```python
from build123d import *

# Parameters (mm, degrees)
SKETCH1_W                = 42
SKETCH1_H                = 14
BOSS_EXTRUDE1_DEPTH      = 20
SKETCH2_W                = 11
SKETCH2_H                = 10
CUT_EXTRUDE1_DEPTH       = 33.202484376
SKETCH3_W                = 11
SKETCH3_H                = 10
CUT_EXTRUDE2_DEPTH       = 33.202484376
SKETCH4_W                = 12
SKETCH4_H                = 10
CUT_EXTRUDE3_DEPTH       = 33.202484376
F_4_0_4_DIAMETER_HOLE1_D = 4
FILLET1_R                = 1
SKETCH7_W                = 53.135320533
SKETCH7_H                = 18.013507302
CUT_EXTRUDE4_DEPTH       = 1.5
SKETCH8_W                = 12
SKETCH8_H                = 12.5
CUT_EXTRUDE5_DEPTH       = 1.5
SKETCH9_W                = 20
SKETCH9_H                = 20
BOSS_EXTRUDE2_DEPTH      = 1
SKETCH10_W               = 3.48641985
SKETCH10_H               = 13.666765812
CUT_EXTRUDE6_DEPTH       = 3
SKETCH11_W               = 4.358024812
SKETCH11_H               = 13.509876918
CUT_EXTRUDE7_DEPTH       = 3
BOSS_EXTRUDE3_START      = 0.5
SKETCH14_W               = 12
SKETCH14_H               = 12.5
SKETCH14_R               = 2
BOSS_EXTRUDE3_DEPTH      = 0.5
FILLET7_R                = 3
BOSS_EXTRUDE4_START      = -14
SKETCH15_W               = 4
SKETCH15_H               = 20
BOSS_EXTRUDE4_DEPTH      = 14
SKETCH16_W               = 13.925462325
SKETCH16_H               = 21.292387115
SKETCH16_W_2             = 9.897316219
SKETCH16_H_2             = 21.744987801
CUT_EXTRUDE8_DEPTH       = 30.241451742
SKETCH17_W               = 12
SKETCH17_H               = 7.5
CUT_EXTRUDE9_DEPTH       = 1.5
SKETCH18_W               = 29.147036291
SKETCH18_H               = 2.174846481
CUT_EXTRUDE10_DEPTH      = 5.897378098
SKETCH19_W               = 12
SKETCH19_H               = 20
BOSS_EXTRUDE5_DEPTH      = 1.5
SKETCH20_W               = 4
SKETCH20_H               = 1.602621902
BOSS_EXTRUDE6_DEPTH      = 1.5
SKETCH24_R               = 1.75
CUT_EXTRUDE11_DEPTH      = 14
SKETCH25_R               = 3.5
CUT_EXTRUDE12_DEPTH      = 1
FILLET8_R                = 2


with BuildPart() as part:
    # Sketch1 → Boss-Extrude1 (new body)
    with BuildSketch(Plane.XZ.offset(6.25)):
        with Locations((0, 7)):
            Rectangle(SKETCH1_W, SKETCH1_H)
    extrude(amount=-BOSS_EXTRUDE1_DEPTH)

    # Sketch2 → Cut-Extrude1 (cut, through all)
    with BuildSketch(Plane(origin=(0, 13.75, 0), x_dir=(-1, 0, 0), z_dir=(0, 1, 0))):
        with Locations((-15.5, 9)):
            Rectangle(SKETCH2_W, SKETCH2_H)
    extrude(amount=-CUT_EXTRUDE1_DEPTH, mode=Mode.SUBTRACT)

    # Sketch3 → Cut-Extrude2 (cut, through all)
    with BuildSketch(Plane(origin=(0, 13.75, 0), x_dir=(-1, 0, 0), z_dir=(0, 1, 0))):
        with Locations((15.5, 9)):
            Rectangle(SKETCH3_W, SKETCH3_H)
    extrude(amount=-CUT_EXTRUDE2_DEPTH, mode=Mode.SUBTRACT)

    # Sketch4 → Cut-Extrude3 (cut, through all)
    with BuildSketch(Plane(origin=(0, 13.75, 0), x_dir=(-1, 0, 0), z_dir=(0, 1, 0))):
        with Locations((0, 5)):
            Rectangle(SKETCH4_W, SKETCH4_H)
    extrude(amount=-CUT_EXTRUDE3_DEPTH, mode=Mode.SUBTRACT)

    # Ø4.0 (4) Diameter Hole1 (through all)
    with Locations(Plane.XY.offset(4)):
        with Locations((15, 0), (-15, 0)):
            Hole(F_4_0_4_DIAMETER_HOLE1_D / 2)

    # Fillet1
    fillet1_edges = [part.edges().sort_by_distance(p)[0] for p in [
        (-21, -6.25, 2),
        (-21, 13.75, 2),
        (21, -6.25, 2),
        (21, 13.75, 2),
    ]]
    fillet(fillet1_edges, radius=FILLET1_R)

    # Sketch7 → Cut-Extrude4 (cut)
    with BuildSketch(Plane(origin=(0, 0, 0), x_dir=(-1, 0, 0), z_dir=(0, 0, -1))):
        with Locations((2.896644391, -1.154131749)):
            Rectangle(SKETCH7_W, SKETCH7_H)
    extrude(amount=-CUT_EXTRUDE4_DEPTH, mode=Mode.SUBTRACT)

    # Sketch8 → Cut-Extrude5 (cut)
    with BuildSketch(Plane(origin=(0, 0, 10), x_dir=(-1, 0, 0), z_dir=(0, 0, -1))):
        Rectangle(SKETCH8_W, SKETCH8_H)
    extrude(amount=-CUT_EXTRUDE5_DEPTH, mode=Mode.SUBTRACT)

    # Sketch9 → Boss-Extrude2 (add)
    with BuildSketch(Plane.XY.offset(14)):
        with Locations((0, 3.75)):
            Rectangle(SKETCH9_W, SKETCH9_H)
    extrude(amount=BOSS_EXTRUDE2_DEPTH)

    # Sketch10 → Cut-Extrude6 (cut)
    with BuildSketch(Plane.ZY.offset(21)):
        with Locations((2.776320836, -0.252765439)):
            Rectangle(SKETCH10_W, SKETCH10_H)
    extrude(amount=-CUT_EXTRUDE6_DEPTH, mode=Mode.SUBTRACT)

    # Sketch11 → Cut-Extrude7 (cut)
    with BuildSketch(Plane(origin=(21, 0, 0), x_dir=(0, 0, -1), z_dir=(1, 0, 0))):
        with Locations((-2.462543049, -0.261481489)):
            Rectangle(SKETCH11_W, SKETCH11_H)
    extrude(amount=-CUT_EXTRUDE7_DEPTH, mode=Mode.SUBTRACT)

    # Sketch14 → Boss-Extrude3 (add)
    # profile 1 of 2: a face of its own
    with BuildSketch(Plane(origin=(0, 0, 1.5), x_dir=(-1, 0, 0), z_dir=(0, 0, -1)).offset(BOSS_EXTRUDE3_START)):
        with Locations((12, 0)):
            Rectangle(SKETCH14_W, SKETCH14_H)
        with Locations(Location((15, 0, 0), (0, 0, 180))):
            Circle(SKETCH14_R, mode=Mode.SUBTRACT)
    # profile 2 of 2: a face of its own
    with BuildSketch(Plane(origin=(0, 0, 1.5), x_dir=(-1, 0, 0), z_dir=(0, 0, -1)).offset(BOSS_EXTRUDE3_START)):
        with Locations((-12, 0)):
            Rectangle(SKETCH14_W, SKETCH14_H)
        with Locations(Location((-15, 0, 0), (0, 0, 180))):
            Circle(SKETCH14_R, mode=Mode.SUBTRACT)
    extrude(amount=-BOSS_EXTRUDE3_DEPTH)

    # Fillet7
    # the kernel refuses this fillet: 3 mm, written as the material it takes off along each edge
    with BuildSketch(Plane(origin=(-18, -6.25, 1.5), x_dir=(1, 0, 0), z_dir=(0, 0, 1))) as fillet7_piece_1:
        with BuildLine():
            CenterArc((FILLET7_R, FILLET7_R), FILLET7_R, 180, 90)
            Line((0, FILLET7_R), (0, 0))
            Line((0, 0), (FILLET7_R, 0))
        make_face()
    extrude(amount=10, mode=Mode.SUBTRACT)
    with BuildSketch(Plane(origin=(18, -6.25, 11.5), x_dir=(-1, 0, 0), z_dir=(0, 0, -1))) as fillet7_piece_2:
        with BuildLine():
            CenterArc((FILLET7_R, FILLET7_R), FILLET7_R, 180, 90)
            Line((0, FILLET7_R), (0, 0))
            Line((0, 0), (FILLET7_R, 0))
        make_face()
    extrude(amount=18, mode=Mode.SUBTRACT)
    with BuildSketch(Plane(origin=(-18, 6.25, -6.5), x_dir=(1, 0, 0), z_dir=(0, 0, 1))) as fillet7_piece_3:
        with BuildLine():
            CenterArc((FILLET7_R, -FILLET7_R), FILLET7_R, 90, 90)
            Line((0, -FILLET7_R), (0, 0))
            Line((0, 0), (FILLET7_R, 0))
        make_face()
    extrude(amount=8, mode=Mode.SUBTRACT)
    with BuildSketch(Plane(origin=(-18, -6.25, -6.5), x_dir=(1, 0, 0), z_dir=(0, 0, 1))) as fillet7_piece_4:
        with BuildLine():
            CenterArc((FILLET7_R, FILLET7_R), FILLET7_R, 180, 90)
            Line((0, FILLET7_R), (0, 0))
            Line((0, 0), (FILLET7_R, 0))
        make_face()
    extrude(amount=8, mode=Mode.SUBTRACT)

    # Sketch15 → Boss-Extrude4 (add)
    with BuildSketch(Plane.XY.offset(15).offset(BOSS_EXTRUDE4_START)):
        with Locations((-12, 3.75)):
            Rectangle(SKETCH15_W, SKETCH15_H)
        with Locations((12, 3.75)):
            Rectangle(SKETCH15_W, SKETCH15_H)
    extrude(amount=BOSS_EXTRUDE4_DEPTH)

    # Sketch16 → Cut-Extrude8 (cut, through all)
    with BuildSketch(Plane.XY.offset(15)):
        with Locations((20.962731162, 3.103806442)):
            Rectangle(SKETCH16_W, SKETCH16_H)
        with Locations((-18.94865811, 2.877506099)):
            Rectangle(SKETCH16_W_2, SKETCH16_H_2)
    extrude(amount=-CUT_EXTRUDE8_DEPTH, mode=Mode.SUBTRACT)

    # Sketch17 → Cut-Extrude9 (cut)
    with BuildSketch(Plane(origin=(0, 0, 10), x_dir=(-1, 0, 0), z_dir=(0, 0, -1))):
        with Locations((0, 10)):
            Rectangle(SKETCH17_W, SKETCH17_H)
    extrude(amount=-CUT_EXTRUDE9_DEPTH, mode=Mode.SUBTRACT)

    # Sketch18 → Cut-Extrude10 (cut)
    with BuildSketch(Plane(origin=(0, 7.852621902, 0), x_dir=(-1, 0, 0), z_dir=(0, -1, 0))):
        with Locations((-0.573518146, 0.087423241)):
            Rectangle(SKETCH18_W, SKETCH18_H)
    extrude(amount=-CUT_EXTRUDE10_DEPTH, mode=Mode.SUBTRACT)

    # Sketch19 → Boss-Extrude5 (add)
    with BuildSketch(Plane(origin=(0, 0, 11.5), x_dir=(-1, 0, 0), z_dir=(0, 0, -1))):
        with Locations((0, 3.75)):
            Rectangle(SKETCH19_W, SKETCH19_H)
    extrude(amount=BOSS_EXTRUDE5_DEPTH)

    # Sketch20 → Boss-Extrude6 (add)
    with BuildSketch(Plane(origin=(0, 0, 1), x_dir=(-1, 0, 0), z_dir=(0, 0, -1))):
        with Locations((-8, 7.051310951)):
            Rectangle(SKETCH20_W, SKETCH20_H)
        with Locations((8, 7.051310951)):
            Rectangle(SKETCH20_W, SKETCH20_H)
    extrude(amount=-BOSS_EXTRUDE6_DEPTH)

    # Sketch24 → Cut-Extrude11 (cut)
    with BuildSketch(Plane(origin=(0, 0, 1), x_dir=(-1, 0, 0), z_dir=(0, 0, -1))):
        with Locations((-10, 5.75)):
            Circle(SKETCH24_R)
        with Locations((10, 5.75)):
            Circle(SKETCH24_R)
    extrude(amount=-CUT_EXTRUDE11_DEPTH, mode=Mode.SUBTRACT)

    # Sketch25 → Cut-Extrude12 (cut)
    with BuildSketch(Plane.XY.offset(15)):
        with Locations((10, 5.75)):
            Circle(SKETCH25_R)
        with Locations((-10, 5.75)):
            Circle(SKETCH25_R)
    extrude(amount=-CUT_EXTRUDE12_DEPTH, mode=Mode.SUBTRACT)

    # Fillet8
    # the kernel refuses this fillet: 2 mm, written as the material it takes off along each edge
    with BuildSketch(Plane(origin=(12, -4.25, 13), x_dir=(0, 0, 1), z_dir=(1, 0, 0))) as fillet8_piece_1_section:
        Polygon((0, 0), (FILLET8_R, 0), (FILLET8_R, FILLET8_R), (0, FILLET8_R), align=None)
    fillet8_piece_1 = extrude(amount=FILLET8_R, mode=Mode.PRIVATE)
    fillet8_piece_1 = fillet8_piece_1 - Plane(origin=(12, -4.25, 13), x_dir=(0, 0.7071067811865475, -0.7071067811865475), z_dir=(1, 0, 0)) * Sphere(FILLET8_R, mode=Mode.PRIVATE)
    add(fillet8_piece_1, mode=Mode.SUBTRACT)
    with BuildSketch(Plane(origin=(-12, -4.25, 13), x_dir=(0, -1, 0), z_dir=(0, 0, 1))) as fillet8_piece_2_section:
        Polygon((0, 0), (FILLET8_R, 0), (FILLET8_R, -FILLET8_R), (0, -FILLET8_R), align=None)
    fillet8_piece_2 = extrude(amount=FILLET8_R, mode=Mode.PRIVATE)
    fillet8_piece_2 = fillet8_piece_2 - Plane(origin=(-12, -4.25, 13), x_dir=(0.7071067811865475, 0.7071067811865475, 0), z_dir=(0, 0, 1)) * Sphere(FILLET8_R, mode=Mode.PRIVATE)
    add(fillet8_piece_2, mode=Mode.SUBTRACT)
    with BuildSketch(Plane(origin=(-12, 11.75, 13), x_dir=(0, 0, 1), z_dir=(0, 1, 0))) as fillet8_piece_3_section:
        Polygon((0, 0), (FILLET8_R, 0), (FILLET8_R, -FILLET8_R), (0, -FILLET8_R), align=None)
    fillet8_piece_3 = extrude(amount=FILLET8_R, mode=Mode.PRIVATE)
    fillet8_piece_3 = fillet8_piece_3 - Plane(origin=(-12, 11.75, 13), x_dir=(0.7071067811865475, 0, -0.7071067811865475), z_dir=(0, 1, 0)) * Sphere(FILLET8_R, mode=Mode.PRIVATE)
    add(fillet8_piece_3, mode=Mode.SUBTRACT)
    with BuildSketch(Plane(origin=(12, 11.75, 13), x_dir=(0, 1, 0), z_dir=(1, 0, 0))) as fillet8_piece_4_section:
        Polygon((0, 0), (FILLET8_R, 0), (FILLET8_R, FILLET8_R), (0, FILLET8_R), align=None)
    fillet8_piece_4 = extrude(amount=FILLET8_R, mode=Mode.PRIVATE)
    fillet8_piece_4 = fillet8_piece_4 - Plane(origin=(12, 11.75, 13), x_dir=(0, -0.7071067811865475, -0.7071067811865475), z_dir=(1, 0, 0)) * Sphere(FILLET8_R, mode=Mode.PRIVATE)
    add(fillet8_piece_4, mode=Mode.SUBTRACT)
    with BuildSketch(Plane(origin=(12, -6.25, 15), x_dir=(0, 1, 0), z_dir=(-1, 0, 0))) as fillet8_piece_5:
        with BuildLine():
            CenterArc((FILLET8_R, FILLET8_R), FILLET8_R, 180, 90)
            Line((0, FILLET8_R), (0, 0))
            Line((0, 0), (FILLET8_R, 0))
        make_face()
    extrude(amount=24, mode=Mode.SUBTRACT)
    with BuildSketch(Plane(origin=(-12, 13.75, 15), x_dir=(0, 0, -1), z_dir=(1, 0, 0))) as fillet8_piece_6:
        with BuildLine():
            CenterArc((FILLET8_R, -FILLET8_R), FILLET8_R, 90, 90)
            Line((0, -FILLET8_R), (0, 0))
            Line((0, 0), (FILLET8_R, 0))
        make_face()
    extrude(amount=24, mode=Mode.SUBTRACT)
    with BuildSketch(Plane(origin=(-14, -6.25, -4), x_dir=(1, 0, 0), z_dir=(0, 0, 1))) as fillet8_piece_7:
        with BuildLine():
            CenterArc((FILLET8_R, FILLET8_R), FILLET8_R, 180, 90)
            Line((0, FILLET8_R), (0, 0))
            Line((0, 0), (FILLET8_R, 0))
        make_face()
    extrude(amount=17, mode=Mode.SUBTRACT)
    with BuildSketch(Plane(origin=(-14, 11.75, 15), x_dir=(1, 0, 0), z_dir=(0, -1, 0)), Plane(origin=(14, 11.75, 15), x_dir=(0, 0, -1), z_dir=(0, -1, 0))) as fillet8_piece_8:
        with BuildLine():
            CenterArc((FILLET8_R, -FILLET8_R), FILLET8_R, 90, 90)
            Line((0, -FILLET8_R), (0, 0))
            Line((0, 0), (FILLET8_R, 0))
        make_face()
    extrude(amount=16, mode=Mode.SUBTRACT)
    with BuildSketch(Plane(origin=(14, -6.25, 13), x_dir=(0, 1, 0), z_dir=(0, 0, -1)), Plane(origin=(14, 13.75, -4), x_dir=(0, -1, 0), z_dir=(0, 0, 1)), Plane(origin=(-14, 13.75, -4), x_dir=(1, 0, 0), z_dir=(0, 0, 1))) as fillet8_piece_9:
        with BuildLine():
            CenterArc((FILLET8_R, -FILLET8_R), FILLET8_R, 90, 90)
            Line((0, -FILLET8_R), (0, 0))
            Line((0, 0), (FILLET8_R, 0))
        make_face()
    extrude(amount=17, mode=Mode.SUBTRACT)


solid = part.part
```
CAD build for the part. Positions are in the model's coordinates, mm. A direction names the side the tool comes from. Round coordinates to 2 decimals unless told otherwise and drop trailing zeros. Order: outer loops, then holes, each group sorted by start corner. A loop starts at its lowest first (then second) coordinate and runs counter-clockwise, first axis right, second up.
Q1. Wall check: L1, parallel to X at y = 3, z = 8; L2, parallel to Y at x = -10, z = 10; L3, parallel to Z at x = 10, y = 3.75. Give the ranges that are in metal, low to high.
Q2. Drop flat-ended pins along their axis: pin 1 (6 mm diameter, centred on x = -1, y = 4.5, fed in from -Z); pin 2 (2 mm diameter, centred on x = -9.5, y = 4.5, fed in from +Z). Give the stop position or say it passes through.
Q3. Two-plate mould, pull along Y, no slides. Class faces 4 (the flat face through (0, 4, 15)), 5 (the flat face through (0, -6.25, 11)), 6 (the flat face through (-12, 5, 14)): pulls with the +Y half, pulls with the -Y half, needs draft (parallel to the pull), parting line crosses it, or undercut.
Q4. Slice it at C-C (y = 5.75). Write the cut outline in (x, z).
Q5. Slice it at B-B (x = -10). Write the cut outline in (y, z).
Q6. Slice it at A-A (z = 4.5). Write the cut outline in (x, y), and give its area (3 significant figures).
Q7. Which spindle directions (+Z, -Z, +X, -X, +Y, -Y) get a long thin tool onto all of the face, cutting with end or side? Do faces 1 (the cylindrical face through (6.503, 5.904, 14.507)), 2 (the flat face through (6, 4, 5)), 3 (the cylindrical face through (0.17, -5.68, 14.4)). Say none if no direction does.
Q8. Slice it at D-D (y = -1). Write the cut outline in (x, z), and give its area (3 significant figures).
Results below:
1. L1: x = -14 to -6, 6 to 14
1. L2: y = -6.25 to 4, 7.5 to 13.75
1. L3: z = 1 to 14
2. pin 1: stops at z = 10
2. pin 2: stops at z = 14
3. face 4: needs draft
3. face 5: pulls with the -Y half
3. face 6: undercut
4. outline: (-14, 1) - (-11.75, 1) - (-11.75, 14) - (-13.5, 14) - (-13.5, 14.32) arc R2 ccw to (-14, 13) - close; (-8.25, 1) - (-6, 1) - (-6, 10) - (6, 10) - (6, 1) - (8.25, 1) - (8.25, 14) - (6.5, 14) - (6.5, 15) - (-6.5, 15) - (-6.5, 14) - (-8.25, 14) - close; (11.75, 1) - (14, 1) - (14, 13) arc R2 ccw to (13.5, 14.32) - (13.5, 14) - (11.75, 14) - close
5. outline: (-6.25, 1) - (4, 1) - (4, 14) - (2.25, 14) - (2.25, 15) - (-4.25, 15) arc R2 ccw to (-6.25, 13) - close; (7.5, 1) - (13.75, 1) - (13.75, 13) arc R2 ccw to (11.75, 15) - (9.25, 15) - (9.25, 14) - (7.5, 14) - close
6. outline: (-14, -4.25) arc R2 ccw to (-12, -6.25) - (-6, -6.25) - (-6, 13.75) - (-12, 13.75) arc R2 ccw to (-14, 11.75) - close; (6, -6.25) - (12, -6.25) arc R2 ccw to (14, -4.25) - (14, 11.75) arc R2 ccw to (12, 13.75) - (6, 13.75) - close; hole circle Ø3.5 at (-10, 5.75); hole circle Ø3.5 at (10, 5.75)
6. area: 297 mm2
7. face 1: +Z
7. face 2: -Z, +Y, -Y
7. face 3: +Z, +X, -X, -Y
8. outline: (-14, 1) - (-6, 1) - (-6, 10) - (6, 10) - (6, 1) - (14, 1) - (14, 13) arc R2 ccw to (12, 15) - (-12, 15) arc R2 ccw to (-14, 13) - close
8. area: 282 mm2
